Design review of the part shown in the three views and the two pictorial views. Dimensions are in mm from the part's minimum x, y and z. A direction names the side the tool comes from. Coordinates: 2 decimals unless noted, no trailing zeros. Write each loop counter-clockwise with the first axis right and the second up, starting at its lowest first coordinate (ties: lowest second). Pieces come first, ordered by that corner, then holes. Notation, with made-up numbers: (9.25, -5) -> (14.25, -5) arc R34 cw to (14.25, 32) -> close; hole circle Ø5 at (41, 70). An arc over 180 degrees is marked (long way). Answer in a Markdown table with one row per item. Add a question column.
Item 1: Take a section at C-C, the plane z = 9.5. Write out the cut boundary in (x, y) (1 decimal).
Item 2: Take a section at A-A, the plane y = 10. Write out the cut boundary in (x, z) (1 decimal).
Item 3: Take a section at D-D, the plane y = 20.5. Write out the cut boundary in (x, z).
Item 4: For the marked faces 1 and 2, list the 3-axis set-ups (+Z, -Z, +X, -X, +Y, -Y) from which the entire face can be reached by the end or side of a thin tool; tool diameter is ignored.
Item 5: Clearance check with flat-ended pins moving along their axes: P1, Ø2, axis at y = 22, z = 16.5, coming from the +X side; P2, Ø3, axis at y = 24, z = 18, coming from the -X side; P3, Ø5, axis at x = 33.5, y = 24, coming from the +Z side; P4, Ø3.5, axis at y = 8.73, z = 28.89, coming from the -X side. State where each tip first meets the part, or that it passes through.
Item 6: To check wall thickness, follow line 1 (X direction, y = 9, z = 25.5). State the ranges of the line that lie inside material, in increasing order.
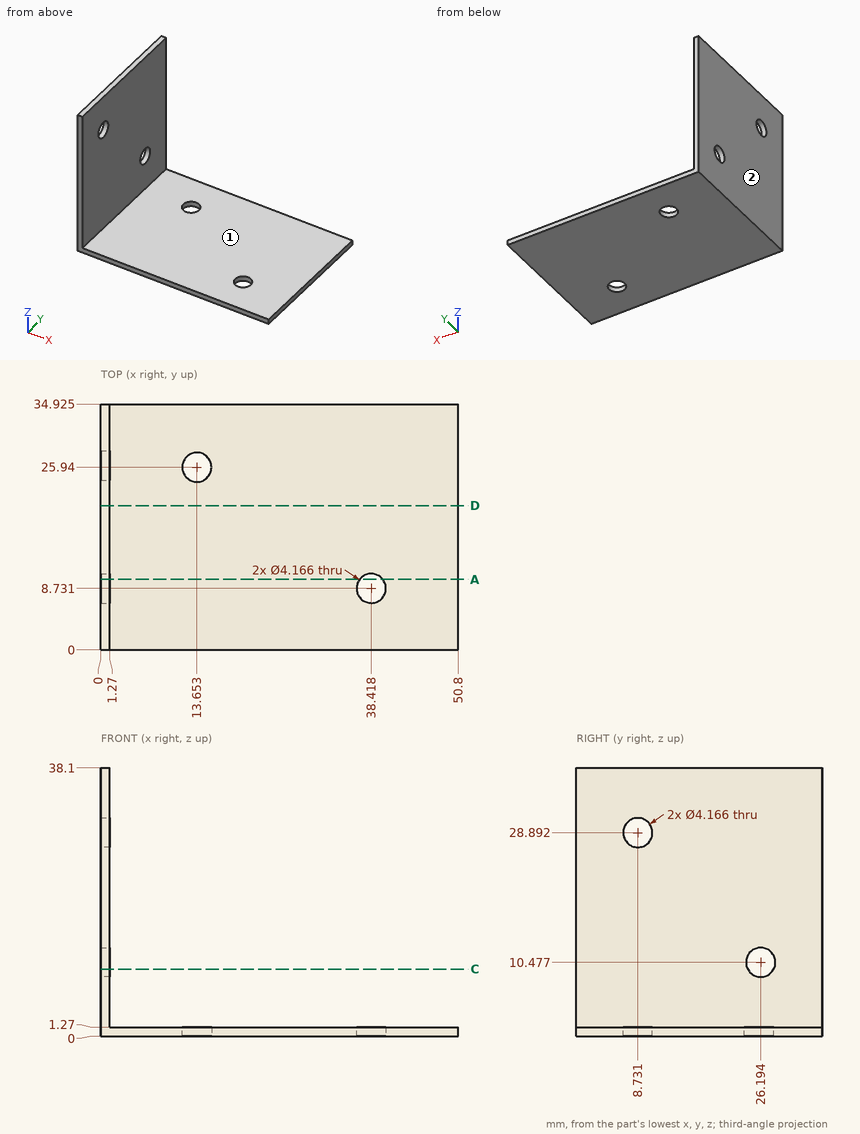
Answers:
| question | item | result |
|---|---|---|
| 1 | outline | (0, 0) -> (1.3, 0) -> (1.3, 24.4) -> (0, 24.4) -> close; (0, 28) -> (1.3, 28) -> (1.3, 34.9) -> (0, 34.9) -> close |
| 2 | outline | (0, 0) -> (36.8, 0) -> (36.8, 1.3) -> (1.3, 1.3) -> (1.3, 27.2) -> (0, 27.2) -> close; (0, 30.5) -> (1.3, 30.5) -> (1.3, 38.1) -> (0, 38.1) -> close; (40.1, 0) -> (50.8, 0) -> (50.8, 1.3) -> (40.1, 1.3) -> close |
| 3 | outline | (0, 0) -> (50.8, 0) -> (50.8, 1.27) -> (1.27, 1.27) -> (1.27, 38.1) -> (0, 38.1) -> close |
| 4 | face 1 | +Z, +X, +Y, -Y |
| 4 | face 2 | +Z, -Z, -X, +Y, -Y |
| 5 | P1 | stops at x = 1.27 |
| 5 | P2 | stops at x = 0 |
| 5 | P3 | stops at z = 1.27 |
| 5 | P4 | passes through |
| 6 | line 1 | x = 0 to 1.27 |
